```python
from build123d import *

# Parameters (mm, degrees)
SKETCH1_W           = 95.25
SKETCH1_H           = 95.25
SKETCH1_R           = 38.1
BOSS_EXTRUDE1_DEPTH = 3.175
FILLET1_R           = 6.35
SKETCH4_R           = 2.159
CUT_EXTRUDE1_DEPTH  = 4.175
FILLET2_R           = 12.7


with BuildPart() as part:
    # Sketch1 → Boss-Extrude1 (new body)
    with BuildSketch(Plane.XY):
        Rectangle(SKETCH1_W, SKETCH1_H)
        Circle(SKETCH1_R, mode=Mode.SUBTRACT)
    extrude(amount=BOSS_EXTRUDE1_DEPTH)

    # Sketch2 → Revolve1 (revolve)
    with BuildSketch(Plane(origin=(0, 0, 0), x_dir=(1, 0, 0), z_dir=(0, 1, 0))):
        Polygon((38.1, -3.175), (38.1, -6.35), (41.275, -3.175), align=None)
    revolve(axis=Axis((0, 0, 1000), (0, 0, -1)))

    # Fillet1
    fillet1_edges = [part.edges().sort_by_distance(p)[0] for p in [
        (-41.275, 0, 3.175),
    ]]
    fillet(fillet1_edges, radius=FILLET1_R)

    # Sketch4 → Cut-Extrude1 (cut, through all)
    with BuildSketch(Plane.XY.offset(3.175)):
        with Locations((-34.925, 34.925)):
            Circle(SKETCH4_R)
        with Locations((34.925, 34.925)):
            Circle(SKETCH4_R)
        with Locations((34.925, -34.925)):
            Circle(SKETCH4_R)
        with Locations((-34.925, -34.925)):
            Circle(SKETCH4_R)
    extrude(amount=-CUT_EXTRUDE1_DEPTH, mode=Mode.SUBTRACT)

    # Fillet2
    fillet2_edges = [part.edges().sort_by_distance(p)[0] for p in [
        (-47.625, 47.625, 1.5875),
        (47.625, 47.625, 1.5875),
        (47.625, -47.625, 1.5875),
        (-47.625, -47.625, 1.5875),
    ]]
    fillet(fillet2_edges, radius=FILLET2_R)


solid = part.part
```
Input: part model. Units: mm. Frame: model coordinates. A direction names the side the tool comes from. Round coordinates to 2 decimals unless told otherwise and drop trailing zeros. Write each loop counter-clockwise with the first axis right and the second up, starting at its lowest first coordinate (ties: lowest second). Pieces come first, ordered by that corner, then holes. Notation, with made-up numbers: M 53.25,48 L 65.25,48 A27 cw 65.25,82 Z; hole C 43.5,-32 d6. An arc over 180 degrees is marked long. Write each question's results on one line, items separated by ' | '.
Q1. Pin query (flat end, axial travel): P1, Ø7, axis at x = -34.925, y = -34.925, coming from the +Z side (3 decimals); P2, Ø1.5, axis at x = -14.5, z = 5, coming from the -Y side; P3, Ø2.5, axis at x = 34.925, y = -34.925, coming from the +Z side. Return the tip coordinate at first contact, or that it passes through.
Results:
P1: stops at z = 3.175 | P2: stops at y = -37.71 | P3: passes through
Q2. Section query A-A (x = 0). Return loops of the section in (y, z) (3 decimals), and give its area (3 significant figures).
Results:
outline: M -47.625,0 L -38.1,0 L -38.1,6.35 L -39.415,5.035 A6.35 cw -43.905,3.175 L -47.625,3.175 Z; M 38.1,0 L 47.625,0 L 47.625,3.175 L 43.905,3.175 A6.35 cw 39.415,5.035 L 38.1,6.35 Z | area: 72.3 mm^2
Q3. Draft query along Y for faces 3 (the face through (43.81, -44, 1.61)), 4 (the face through (36.086, -33.105, 1.61)), 5 (the face through (-47.625, 0, 2)). Return one class per face: released by +Y, released by -Y, zero draft, split by the parting line, or undercut.
Results:
face 3: released by -Y | face 4: undercut | face 5: zero draft
Q4. Section query C-C (z = 2). Return loops of the section in (x, y) (3 decimals), and give its area (3 significant figures).
Results:
outline: M -47.625,-34.925 A12.7 ccw -34.925,-47.625 L 34.925,-47.625 A12.7 ccw 47.625,-34.925 L 47.625,34.925 A12.7 ccw 34.925,47.625 L -34.925,47.625 A12.7 ccw -47.625,34.925 Z; hole C 0,0 d76.2; hole C -34.925,-34.925 d4.318; hole C -34.925,34.925 d4.318; hole C 34.925,-34.925 d4.318; hole C 34.925,34.925 d4.318 | area: 4,320 mm^2
Q5. Access query for faces 1 (the face through (-35.206, 37.066, 1.61)), 2 (the face through (-11, 43, 3.175)). Directions: +Z, -Z, +X, -X, +Y, -Y. A direction counts if a zero-diameter tool reaches every point of the face in a straight line with its end or side. Return the directions, or none.
Results:
face 1: +Z, -Z | face 2: +Z
Q6. Line query: line 1 along X through (y, z) = (34, 1.75) (3 decimals); line 2 along X through (y, z) = (0, 2) (3 decimals); line 3 along Z through (x, y) = (37, 32.5) (3 decimals). Output: solid intervals per line, ascending.
Results:
line 1: x = -47.625 to -36.876, -32.974 to -17.193, 17.193 to 32.974, 36.876 to 47.625 | line 2: x = -47.625 to -38.1, 38.1 to 47.625 | line 3: z = 0 to 3.175
